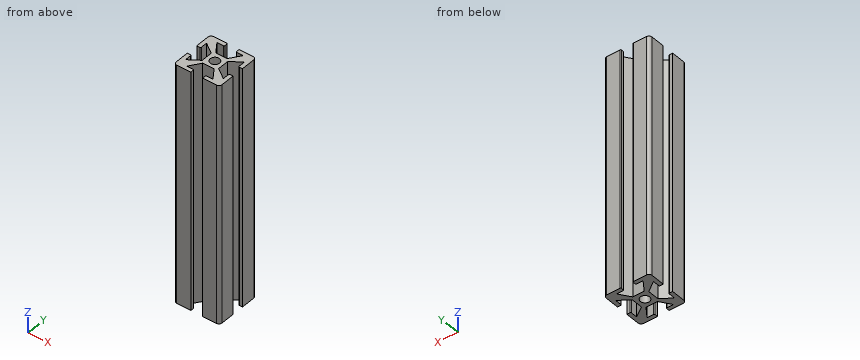
```python
from build123d import *

# Parameters (mm, degrees)
SKETCH1_W           = 25.4
SKETCH1_H           = 25.4
BOSS_EXTRUDE1_DEPTH = 132.588
FILLET1_R           = 1.5875
HOLE1_OUTLINE_R     = 2.5527
HOLE1_DEPTH         = 132.588
SKETCH7_W           = 6.5278
SKETCH7_H           = 2.2352
CUT_EXTRUDE2_DEPTH  = 132.588
FILLET4_R           = 0.396875
CIRPATTERN2_DEPTH   = 132.588


# Read off the part's stored shape, not the designer's step: Hole1, CirPattern2
with BuildPart() as part:
    # Sketch1 → Boss-Extrude1 (new body)
    with BuildSketch(Plane.XY):
        Rectangle(SKETCH1_W, SKETCH1_H)
    extrude(amount=BOSS_EXTRUDE1_DEPTH)

    # Fillet1
    fillet1_edges = [part.edges().sort_by_distance(p)[0] for p in [
        (12.7, -12.7, 66.294),
        (-12.7, -12.7, 66.294),
        (-12.7, 12.7, 66.294),
        (12.7, 12.7, 66.294),
    ]]
    fillet(fillet1_edges, radius=FILLET1_R)

    # Hole1 outline → Hole1 (cut)
    with BuildSketch(Plane.XY):
        with Locations((0, -0.048792482)):
            Circle(HOLE1_OUTLINE_R)
    extrude(amount=HOLE1_DEPTH, mode=Mode.SUBTRACT)

    # Sketch7 → Cut-Extrude2 (cut)
    with BuildSketch(Plane.XY.offset(132.588)):
        with Locations((0, 11.5824)):
            Rectangle(SKETCH7_W, SKETCH7_H)
        Polygon((-3.175, 4.5212), (-7.3025, 10.4648), (7.3025, 10.4648), (3.175, 4.5212), align=None)
    extrude(amount=-CUT_EXTRUDE2_DEPTH, mode=Mode.SUBTRACT)

    # Fillet4
    fillet4_edges = [part.edges().sort_by_distance(p)[0] for p in [
        (-3.2639, 10.4648, 66.294),
        (-3.2639, 12.7, 66.294),
        (3.2639, 12.7, 66.294),
        (3.2639, 10.4648, 66.294),
    ]]
    fillet(fillet4_edges, radius=FILLET4_R)

    # CirPattern2 outline → CirPattern2 (cut)
    with BuildSketch(Plane.XY):
        with BuildLine():
            ThreePointArc((-3.660775, -10.562384964), (-3.380141996, -10.67862696), (-3.2639, -10.959259964))
            Line((-3.2639, -10.959259964), (-3.2639, -12.7))
            Line((-3.2639, -12.7), (3.2639, -12.7))
            Line((3.2639, -12.7), (3.2639, -10.959259964))
            ThreePointArc((3.2639, -10.959259964), (3.380141996, -10.67862696), (3.660775, -10.562384964))
            Line((3.660775, -10.562384964), (7.3025, -10.562384964))
            Line((7.3025, -10.562384964), (3.175, -4.618784964))
            Line((3.175, -4.618784964), (-3.175, -4.618784964))
            Line((-3.175, -4.618784964), (-7.3025, -10.562384964))
            Line((-7.3025, -10.562384964), (-3.660775, -10.562384964))
        make_face()
        with BuildLine():
            Line((-12.7, -3.312692482), (-10.910467482, -3.312692482))
            ThreePointArc((-10.910467482, -3.312692482), (-10.629834478, -3.428934478), (-10.513592482, -3.709567482))
            Line((-10.513592482, -3.709567482), (-10.513592482, -7.351292482))
            Line((-10.513592482, -7.351292482), (-4.569992482, -3.223792482))
            Line((-4.569992482, -3.223792482), (-4.569992482, 3.126207518))
            Line((-4.569992482, 3.126207518), (-10.513592482, 7.253707518))
            Line((-10.513592482, 7.253707518), (-10.513592482, 3.611982518))
            ThreePointArc((-10.513592482, 3.611982518), (-10.629834478, 3.331349514), (-10.910467482, 3.215107518))
            Line((-10.910467482, 3.215107518), (-12.7, 3.215107518))
            Line((-12.7, 3.215107518), (-12.7, -3.312692482))
        make_face()
        with BuildLine():
            ThreePointArc((10.513592482, -3.709567482), (10.629834478, -3.428934478), (10.910467482, -3.312692482))
            Line((10.910467482, -3.312692482), (12.7, -3.312692482))
            Line((12.7, -3.312692482), (12.7, 3.215107518))
            Line((12.7, 3.215107518), (10.910467482, 3.215107518))
            ThreePointArc((10.910467482, 3.215107518), (10.629834478, 3.331349514), (10.513592482, 3.611982518))
            Line((10.513592482, 3.611982518), (10.513592482, 7.253707518))
            Line((10.513592482, 7.253707518), (4.569992482, 3.126207518))
            Line((4.569992482, 3.126207518), (4.569992482, -3.223792482))
            Line((4.569992482, -3.223792482), (10.513592482, -7.351292482))
            Line((10.513592482, -7.351292482), (10.513592482, -3.709567482))
        make_face()
    extrude(amount=CIRPATTERN2_DEPTH, mode=Mode.SUBTRACT)


solid = part.part
```
Geometry: final body of the model. Coordinates: model frame, mm. Coordinates: 2 decimals unless noted, no trailing zeros. Write each loop counter-clockwise with the first axis right and the second up, starting at its lowest first coordinate (ties: lowest second). Pieces come first, ordered by that corner, then holes. Notation, with made-up numbers: M -21.75,70.25 L -8.75,70.25 A36 ccw -8.75,106.25 Z; hole C 24,-4 d6. An arc over 180 degrees is marked long. Answer as CSV lines item,"result". Start each with the question number.
Q1. Cut plane A-A on x = 0. Return the cut outline in (y, z).
Q2. Pin query (flat end, axial travel): P1, Ø0.5, axis at x = 12, z = 39.5, coming from the -Y side; P2, Ø1.9, axis at x = -0.5, z = 85, coming from the -Y side; P3, Ø0.5, axis at x = -11.5, z = 61.5, coming from the +Y side. Return the tip coordinate at first contact, or that it passes through.
Q3. Line query: line 1 (X direction, y = -3.5, z = 85); line 2 (X direction, y = 11.25, z = 54); line 3 (X direction, y = 5.75, z = 75). Output: solid intervals per line, ascending. Write a range as from..to.
Q4. Cut plane B-B on y = -8.75. Return the cut outline in (x, z).
Findings below:
1,outline,"M -4.62,0 L -2.6,0 L -2.6,132.59 L -4.62,132.59 Z; M 2.5,0 L 4.52,0 L 4.52,132.59 L 2.5,132.59 Z"
2,P1,"stops at y = -12.57"
2,P2,"stops at y = -4.62"
2,P3,"stops at y = 12.69"
3,line 1,"x = -12.7..-10.57, -4.97..4.97, 10.57..12.7"
3,line 2,"x = -12.69..-3.26, 3.26..12.69"
3,line 3,"x = -12.7..-10.51, -8.35..-4.03, 4.03..8.35, 10.51..12.7"
4,outline,"M -12.7,0 L -6.04,0 L -6.04,132.59 L -12.7,132.59 Z; M 6.04,0 L 12.7,0 L 12.7,132.59 L 6.04,132.59 Z"
